from build123d import *

# Parameters (mm, degrees)
F1_DEPTH = 15
F2_D     = 31


with BuildPart() as f1:
    # F0 (on Front) → F1 (new body)
    with BuildSketch(Plane.XZ):
        with BuildLine():
            ThreePointArc((-65.015006, 48.24327), (-96.069918, 0), (-65.015006, -48.24327))
            Line((-65.015006, -48.24327), (97.984994, -48.24327))
            Line((97.984994, -48.24327), (109.984994, 48.24327))
            Line((109.984994, 48.24327), (-65.015006, 48.24327))
        make_face()
    extrude(amount=F1_DEPTH)

    # F2 (through all)
    with Locations(Plane(origin=(0, 0, 0), x_dir=(1, 0, 0), z_dir=(0, 1, 0))):
        with Locations((-52.069918, 0)):
            Hole(F2_D / 2)


solid = f1.part
Work out the finished part from the listing and answer in its coordinate system (mm). Coordinates: 2 decimals unless noted, no trailing zeros. Write each loop counter-clockwise with the first axis right and the second up, starting at its lowest first coordinate (ties: lowest second). Pieces come first, ordered by that corner, then holes. Notation, with made-up numbers: M 44.5,65 L 52.5,65 A17 ccw 52.5,97 Z; hole C -7,71.5 d11. An arc over 180 degrees is marked long. Use one line per item in the form item = value. Start each with the question number.
1. The part is cut by section A-A (y = -6). Give the vertices of the cut face in (x, z) (3 decimals).
2. The mould has two halves that part along X. Classify faces 1 (the face through (103.9, -7.4, -0.68)), 2 (the face through (-96.063, -7.395, 0.849)), 3 (the face through (6, -15, 1)), 4 (the face through (-66.854, -7.605, -4.656)): released by +X, released by -X, zero draft, split by the parting line, or undercut.
3. The part is cut by section B-B (x = -51.5). Give the vertices of the cut face in (y, z).
4. The part is cut by section C-C (z = 0). Give the vertices of the cut face in (x, y) (3 decimals), plus the area to 3 significant figures.
5. The part is cut by section D-D (z = -27.5). Give the vertices of the cut face in (x, y).
6. Each of these flat-tipped pins is pushed along its axis until it touches: P1, Ø6, axis at y = -12.5, z = -15, coming from the -X side; P2, Ø4, axis at y = -11, z = -9, coming from the +X side. Where does it stop, or does it pass through?
7. Straight lines are drawn through the part: probe 1 along Z at (x, y) = (-52, -2.25); probe 2 along Z at (x, y) = (-54, -5.25); probe 3 along X at (y, z) = (-12.25, 7). For each, find the intervals that lie inside material, in ascending order. Write a range as from..to.
Evaluation:
q1.outline = M -65.015,-48.243 L 97.985,-48.243 L 109.985,48.243 L -65.015,48.243 A53 ccw Z; hole C -52.07,0 d31
q2.face_1 = released by +X
q2.face_2 = released by -X
q2.face_3 = zero draft
q2.face_4 = undercut
q3.outline = M -15,-48.24 L 0,-48.24 L 0,-15.49 L -15,-15.49 Z; M -15,15.49 L 0,15.49 L 0,48.24 L -15,48.24 Z
q4.outline = M -96.07,-15 L -67.57,-15 L -67.57,0 L -96.07,0 Z; M -36.57,-15 L 103.985,-15 L 103.985,0 L -36.57,0 Z
q4.area = 2,540 mm^2
q5.outline = M -88.38,-15 L 100.56,-15 L 100.56,0 L -88.38,0 Z
q6.P1 = -94.69
q6.P2 = 103.11
q7.probe_1 = -48.24..-15.5, 15.5..48.24
q7.probe_2 = -48.24..-15.38, 15.38..48.24
q7.probe_3 = -95.61..-65.9, -38.24..104.86
